Source: three-view drawing plus pictorial views. Frame: mm from the lowest corner of the part. Round coordinates to 2 decimals unless told otherwise and drop trailing zeros. Write each loop counter-clockwise with the first axis right and the second up, starting at its lowest first coordinate (ties: lowest second). Pieces come first, ordered by that corner, then holes. Notation, with made-up numbers: M 86,21.25 L 98,21.25 A29 ccw 98,48.25 Z; hole C 76,74 d3. An arc over 180 degrees is marked long. Answer as CSV lines item,"result". Start each with the question number.
Q1. Section query C-C on y = 1.35. Give the number of separate pieces and of enclosed holes in the cut face, and give its area (3 significant figures).
Q2. Section query A-A on x = 155.5. Output: boundary loops of the cut face in (y, z) (1 decimal).
Q3. Section query B-B on z = 42.5. Output: boundary loops of the cut face in (x, y) (1 decimal).
Q4. Ray query, probe 1 along X at (y, z) = (1.65, 95.75) (1 decimal); probe 2 along Z at (x, y) = (153, 0.85); probe 3 along X at (y, z) = (1.8, 87) (1 decimal). Return the intervals inside material, ascending.
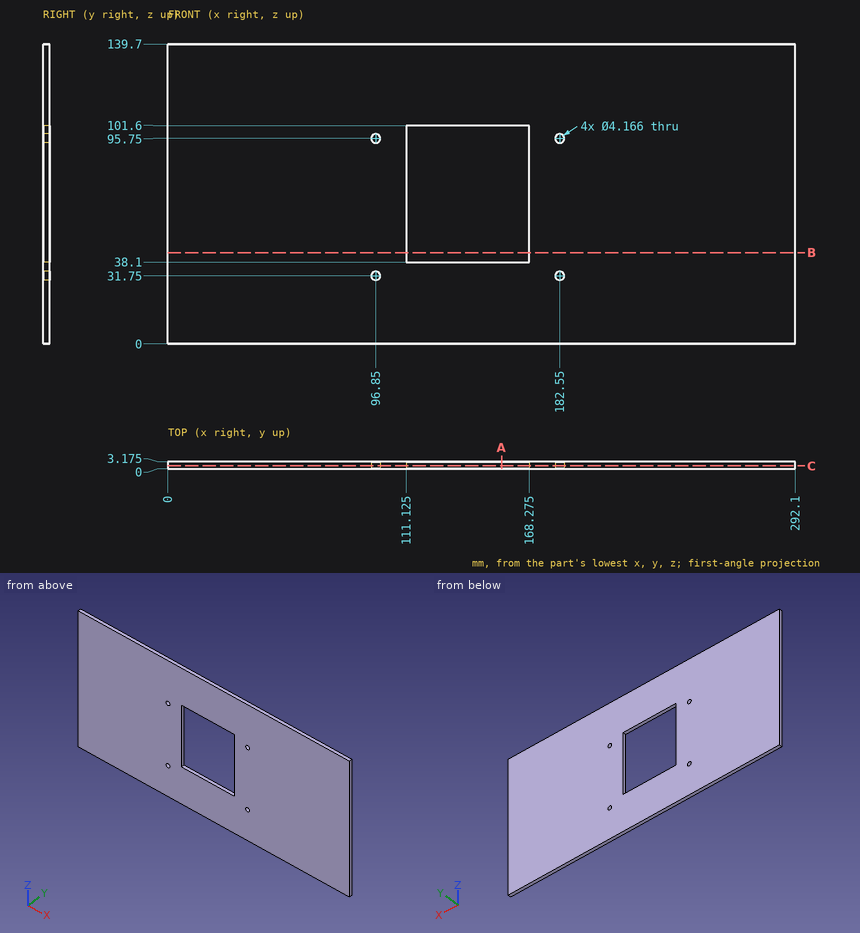
Entries:
1,separate pieces,"1"
1,enclosed holes,"5"
1,area,"37,100 mm^2"
2,outline,"M 0,0 L 3.2,0 L 3.2,38.1 L 0,38.1 Z; M 0,101.6 L 3.2,101.6 L 3.2,139.7 L 0,139.7 Z"
3,outline,"M 0,0 L 111.1,0 L 111.1,3.2 L 0,3.2 Z; M 168.3,0 L 292.1,0 L 292.1,3.2 L 168.3,3.2 Z"
4,probe 1,"x = 0 to 94.8, 98.9 to 111.1, 168.3 to 180.5, 184.6 to 292.1"
4,probe 2,"z = 0 to 38.1, 101.6 to 139.7"
4,probe 3,"x = 0 to 111.1, 168.3 to 292.1"
